```python
from build123d import *

# Parameters (mm, degrees)
CYLINDER116_R              = 8.5
CYLINDER116_DEPTH          = 3
CYLINDER115_R              = 10
CYLINDER115_DEPTH          = 3
CYLINDER110_R              = 0.8
CYLINDER110_DEPTH          = 20
CYLINDER107_R              = 0.8
CYLINDER107_DEPTH          = 20
FUSION028_PLACEMENT_ANGLE  = 54
CYLINDER112_R              = 0.8
CYLINDER112_DEPTH          = 20
CYLINDER111_R              = 0.8
CYLINDER111_DEPTH          = 20
FUSION106_PLACEMENT_ANGLE  = 162
CYLINDER114_R              = 0.8
CYLINDER114_DEPTH          = 20
CYLINDER113_R              = 0.8
CYLINDER113_DEPTH          = 20
FUSION107_PLACEMENT_ANGLE  = 126
CYLINDER106_R              = 0.8
CYLINDER106_DEPTH          = 20
CYLINDER105_R              = 0.8
CYLINDER105_DEPTH          = 20
FUSION108_PLACEMENT_ANGLE  = 90
CYLINDER108_R              = 0.8
CYLINDER108_DEPTH          = 20
CYLINDER104_R              = 0.8
CYLINDER104_DEPTH          = 20
FUSION105_PLACEMENT_ANGLE  = 18
CYLINDER062_R              = 3
CYLINDER062_DEPTH          = 4
CYLINDER061_R              = 5.6
CYLINDER061_DEPTH          = 4
CYLINDER060_R              = 5.6
CYLINDER060_DEPTH          = 4
CYLINDER103_R              = 7
CYLINDER103_DEPTH          = 1.5
CYLINDER109_R              = 10
CYLINDER109_DEPTH          = 6
CYLINDER058_R              = 15
CYLINDER058_DEPTH          = 6
CHAMFER002_SIZE            = 1
CHAMFER002_PLACEMENT_ANGLE = 90


with BuildPart() as cylinder116:
    # Cylinder116 → Cylinder116 (new body)
    with BuildSketch(Plane.XY.offset(11)):
        Circle(CYLINDER116_R)
    extrude(amount=CYLINDER116_DEPTH)


with BuildPart() as cut037:
    # Cylinder115 → Cylinder115 (new body)
    with BuildSketch(Plane.XY.offset(11)):
        Circle(CYLINDER115_R)
    extrude(amount=CYLINDER115_DEPTH)

    # Cut037: cut Cylinder116
    add(cylinder116.part, mode=Mode.SUBTRACT)


with BuildPart() as cylinder110:
    # Cylinder110 → Cylinder110 (new body)
    with BuildSketch(Plane(origin=(-12.5, 0, 13), x_dir=(1, 0, 0), z_dir=(0, 0, 1))):
        Circle(CYLINDER110_R)
    extrude(amount=CYLINDER110_DEPTH)


with BuildPart() as fusion028:
    # Cylinder107 → Cylinder107 (new body)
    with BuildSketch(Plane(origin=(12.5, 0, 13), x_dir=(1, 0, 0), z_dir=(0, 0, 1))):
        Circle(CYLINDER107_R)
    extrude(amount=CYLINDER107_DEPTH)

    # Fusion028: union Cylinder110
    add(cylinder110.part)


with BuildPart() as fusion028_1:
    # Fusion028 placement: moved
    add(fusion028.part.rotate(Axis((0, 0, 0), (0, 0, 1)), FUSION028_PLACEMENT_ANGLE))


with BuildPart() as cylinder112:
    # Cylinder112 → Cylinder112 (new body)
    with BuildSketch(Plane(origin=(-12.5, 0, 13), x_dir=(1, 0, 0), z_dir=(0, 0, 1))):
        Circle(CYLINDER112_R)
    extrude(amount=CYLINDER112_DEPTH)


with BuildPart() as fusion106:
    # Cylinder111 → Cylinder111 (new body)
    with BuildSketch(Plane(origin=(12.5, 0, 13), x_dir=(1, 0, 0), z_dir=(0, 0, 1))):
        Circle(CYLINDER111_R)
    extrude(amount=CYLINDER111_DEPTH)

    # Fusion106: union Cylinder112
    add(cylinder112.part)


with BuildPart() as fusion106_1:
    # Fusion106 placement: moved
    add(fusion106.part.rotate(Axis((0, 0, 0), (0, 0, 1)), FUSION106_PLACEMENT_ANGLE))


with BuildPart() as cylinder114:
    # Cylinder114 → Cylinder114 (new body)
    with BuildSketch(Plane(origin=(-12.5, 0, 13), x_dir=(1, 0, 0), z_dir=(0, 0, 1))):
        Circle(CYLINDER114_R)
    extrude(amount=CYLINDER114_DEPTH)


with BuildPart() as fusion107:
    # Cylinder113 → Cylinder113 (new body)
    with BuildSketch(Plane(origin=(12.5, 0, 13), x_dir=(1, 0, 0), z_dir=(0, 0, 1))):
        Circle(CYLINDER113_R)
    extrude(amount=CYLINDER113_DEPTH)

    # Fusion107: union Cylinder114
    add(cylinder114.part)


with BuildPart() as fusion107_1:
    # Fusion107 placement: moved
    add(fusion107.part.rotate(Axis((0, 0, 0), (0, 0, 1)), FUSION107_PLACEMENT_ANGLE))


with BuildPart() as cylinder106:
    # Cylinder106 → Cylinder106 (new body)
    with BuildSketch(Plane(origin=(-12.5, 0, 13), x_dir=(1, 0, 0), z_dir=(0, 0, 1))):
        Circle(CYLINDER106_R)
    extrude(amount=CYLINDER106_DEPTH)


with BuildPart() as fusion108:
    # Cylinder105 → Cylinder105 (new body)
    with BuildSketch(Plane(origin=(12.5, 0, 13), x_dir=(1, 0, 0), z_dir=(0, 0, 1))):
        Circle(CYLINDER105_R)
    extrude(amount=CYLINDER105_DEPTH)

    # Fusion108: union Cylinder106
    add(cylinder106.part)


with BuildPart() as fusion108_1:
    # Fusion108 placement: moved
    add(fusion108.part.rotate(Axis((0, 0, 0), (0, 0, 1)), FUSION108_PLACEMENT_ANGLE))


with BuildPart() as cylinder108:
    # Cylinder108 → Cylinder108 (new body)
    with BuildSketch(Plane(origin=(-12.5, 0, 13), x_dir=(1, 0, 0), z_dir=(0, 0, 1))):
        Circle(CYLINDER108_R)
    extrude(amount=CYLINDER108_DEPTH)


with BuildPart() as fusion109:
    # Cylinder104 → Cylinder104 (new body)
    with BuildSketch(Plane(origin=(12.5, 0, 13), x_dir=(1, 0, 0), z_dir=(0, 0, 1))):
        Circle(CYLINDER104_R)
    extrude(amount=CYLINDER104_DEPTH)

    # Fusion105: union Cylinder108
    add(cylinder108.part)


with BuildPart() as fusion109_1:
    # Fusion105 placement: moved
    add(fusion109.part.rotate(Axis((0, 0, 0), (0, 0, 1)), FUSION105_PLACEMENT_ANGLE))

    # Fusion109: union Fusion028, Fusion106, Fusion107, Fusion108
    add(fusion028_1.part)
    add(fusion106_1.part)
    add(fusion107_1.part)
    add(fusion108_1.part)


with BuildPart() as fusion109_2:
    # Fusion109 placement: moved
    add(fusion109_1.part.moved(Location((0, 0, 3))))


with BuildPart() as cylinder062:
    # Cylinder062 → Cylinder062 (new body)
    with BuildSketch(Plane.XY.offset(3)):
        Circle(CYLINDER062_R)
    extrude(amount=CYLINDER062_DEPTH)


with BuildPart() as cylinder061:
    # Cylinder061 → Cylinder061 (new body)
    with BuildSketch(Plane.XY):
        Circle(CYLINDER061_R)
    extrude(amount=CYLINDER061_DEPTH)


with BuildPart() as fusion033:
    # Cylinder060 → Cylinder060 (new body)
    with BuildSketch(Plane.XY.offset(6.5)):
        Circle(CYLINDER060_R)
    extrude(amount=CYLINDER060_DEPTH)

    # Fusion033: union Cylinder062, Cylinder061
    add(cylinder062.part)
    add(cylinder061.part)


with BuildPart() as fusion033_1:
    # Fusion033 placement: moved
    add(fusion033.part.moved(Location((0, 0, 4.5))))


with BuildPart() as cylinder103:
    # Cylinder103 → Cylinder103 (new body)
    with BuildSketch(Plane.XY.offset(3)):
        Circle(CYLINDER103_R)
    extrude(amount=CYLINDER103_DEPTH)


with BuildPart() as cylinder109:
    # Cylinder109 → Cylinder109 (new body)
    with BuildSketch(Plane.XY.offset(3)):
        Circle(CYLINDER109_R)
    extrude(amount=CYLINDER109_DEPTH)


with BuildPart() as hub_wide_left:
    # Cylinder058 → Cylinder058 (new body)
    with BuildSketch(Plane.XY.offset(9)):
        Circle(CYLINDER058_R)
    extrude(amount=CYLINDER058_DEPTH)

    # Fusion110: union Cylinder109
    add(cylinder109.part)

    # Cut034: cut Cylinder103
    add(cylinder103.part, mode=Mode.SUBTRACT)

    # Cut035: cut Fusion033
    add(fusion033_1.part, mode=Mode.SUBTRACT)


with BuildPart() as hub_wide_left_1:
    # Cut035 placement: moved
    add(hub_wide_left.part.moved(Location((0, 0, 8))))

    # Cut036: cut Fusion109
    add(fusion109_2.part, mode=Mode.SUBTRACT)

    # Cut038: cut Cut037
    add(cut037.part, mode=Mode.SUBTRACT)

    # Chamfer002
    chamfer002_edges = [hub_wide_left_1.edges().sort_by_distance(p)[0] for p in [
        (-15, 0, 23),
    ]]
    chamfer(chamfer002_edges, length=CHAMFER002_SIZE)


with BuildPart() as hub_wide_left_2:
    # Chamfer002 placement: moved
    add(hub_wide_left_1.part.moved(Location((0, -88, 0))).rotate(Axis((0, -88, 0), (-1, 0, 0)), CHAMFER002_PLACEMENT_ANGLE))


solid = hub_wide_left_2.part
```
Could you check a few things on this model? Use its own coordinates, in mm. A direction names the side the tool comes from. Coordinates: 2 decimals unless noted, no trailing zeros. Answer as CSV lines item,"result". Start each with the question number.
1) For faces 4 (the flat face through (2.4, -69, 2.4)), 5 (the flat face through (2.4, -71.5, 2.4)), 6 (the cylindrical face through (12.64, -68.04, 4.14)), which set-ups out of +Z, -Z, +X, -X, +Y, -Y let a thin tool reach every point of the face, with its end or its side?
2) Please list where these lines run through material, in increasing order: line 1 (X direction, y = -67.75, z = 3.75); line 2 (Z direction, x = -11.75, y = -66.5); line 3 (Z direction, x = -0.5, y = -68). Write a range as from..to.
3) I want a section at B-B, the plane x = 0. Give the number of separate pieces and of enclosed holes in the cut face, and give its area (3 significant figures).
4) For P1, Ø3.5, axis at x = -2.5, z = 0.5, coming from the +Y side; P2, Ø8, axis at x = 0, z = 0, coming from the -Y side; P3, Ø2.5, axis at x = 0, z = -12.5, coming from the -Y side, each with a flat end and sliding along its axis, tell me the tip position at first contact or that it passes through.
5) We'd pull the mould along X, two halves only. Please class faces 1 (the cylindrical face through (4.614, -72.521, 8.872)), 2 (the cylindrical face through (6.466, -76.261, 2.681)), 3 (the flat face through (-4.5, -74, 7.4)): +X half, -X half, draft (parallel to the pull), parting line (faces both ways), or undercut.
Data:
1,face 4,"+Y"
1,face 5,"-Y"
1,face 6,"+Y, -Y"
2,line 1,"x = -14.52..-12.68, -11.1..-4.16, 4.16..11.1, 12.68..14.52"
2,line 2,"z = -9.32..-4.65, -3.07..3.07, 4.65..9.32"
2,line 3,"z = -14.99..-13.12, -11.88..-5.58, 5.58..11.88, 13.12..14.99"
3,separate pieces,"4"
3,enclosed holes,"0"
3,area,"145 mm^2"
4,P1,"stops at y = -69"
4,P2,"stops at y = -71.5"
4,P3,"stops at y = -71"
5,face 1,"parting line"
5,face 2,"undercut"
5,face 3,"draft"
